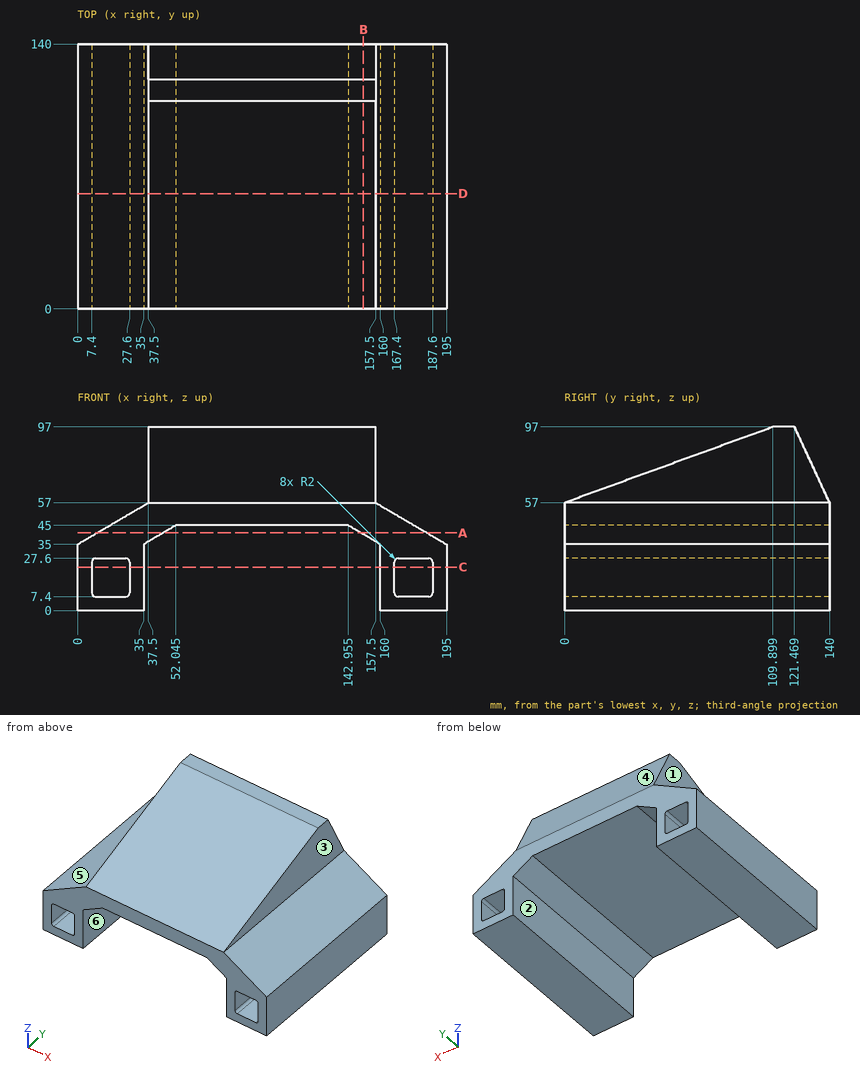
Could you check a few things on this drawing? It's one solid part, dimensions in mm from its lowest x, y, z. A direction names the side the tool comes from. Coordinates: 2 decimals unless noted, no trailing zeros. Order: outer loops, then holes, each group sorted by start corner. A loop starts at its lowest first (then second) coordinate and runs counter-clockwise, first axis right, second up. Notation, with made-up numbers: (83.5, 30.25) - (126.5, 30.25) arc R18 cw to (126.5, 43.25) - close; hole circle Ø3 at (-5, 62). An arc over 180 degrees is marked (long way). One line per question, with ' | ' between items. Start each with the question number.
1. Please list where these lines run through material, in increasing order: line 1 along X through (y, z) = (100.5, 34.5); line 2 along Z through (x, y) = (182, 9.5) (1 decimal); line 3 along X through (y, z) = (82, 68.5). Write a range as [from, to].
2. If we mould it in two halves opening along X, with no side actions, what happens to the marked faces 4, 5 and 6? For each: released by +X, released by -X, zero draft, split by the parting line, or undercut.
3. If we section it at B-B (x = 151): Write out the boundary of the cut face in (y, z).
4. If we section it at C-C (z = 23): Write out the boundary of the cut face in (x, y).
5. Which directions (+Z, -Z, +X, -X, +Y, -Y) give clear straight access to the entire face, cutting with the end or side of a thin tool? Please do the marked faces 1, 2 and 3.
6. If we section it at A-A (z = 41): Write out the boundary of the cut face in (x, y), and give its area (3 significant figures).
7. If we section it at D-D (y = 61): Give the number of separate pieces and of enclosed holes in the cut face, and give its area (3 significant figures).
8. I'm going to push flat-ended pins straight in: pin 1 Ø6 at (x, y) = (152.5, 108.5) entering from -Z; pin 2 Ø4 at (x, y) = (156.5, 60) entering from +Z; pin 3 Ø1 at (x, y) = (61, 100) entering from -Z. Where does each tip first touch, or does it pass through?
Model answer:
1) line 1: x = [0, 35], [160, 195] | line 2: z = [0, 7.4], [27.6, 42.6] | line 3: x = [37.5, 157.5]
2) face 4: zero draft | face 5: released by -X | face 6: undercut
3) outline: (0, 40.28) - (140, 40.28) - (140, 57) - (121.47, 97) - (109.9, 97) - (0, 57) - close
4) outline: (0, 0) - (7.4, 0) - (7.4, 140) - (0, 140) - close; (27.6, 0) - (35, 0) - (35, 140) - (27.6, 140) - close; (160, 0) - (167.4, 0) - (167.4, 140) - (160, 140) - close; (187.6, 0) - (195, 0) - (195, 140) - (187.6, 140) - close
5) face 1: +Z, -X, +Y, -Y | face 2: -Z, +Y, -Y | face 3: +Z, +X, +Y, -Y
6) outline: (10.23, 0) - (45.23, 0) - (45.23, 140) - (10.23, 140) - close; (149.77, 0) - (184.77, 0) - (184.77, 140) - (149.77, 140) - close | area: 9,800 mm²
7) separate pieces: 1 | enclosed holes: 2 | area: 6,690 mm²
8) pin 1: stops at z = 37.64 | pin 2: stops at z = 79.57 | pin 3: stops at z = 45
